Input: dimensioned drawing with shaded views. Units: mm. Origin: part minimum x, y, z. Give positions to 0.01 mm unless a question says otherwise; leave off trailing zeros. Loops run counter-clockwise (first coordinate to the right, second up) from the corner with the lowest first, then second, coordinate; pieces in that order, holes last.
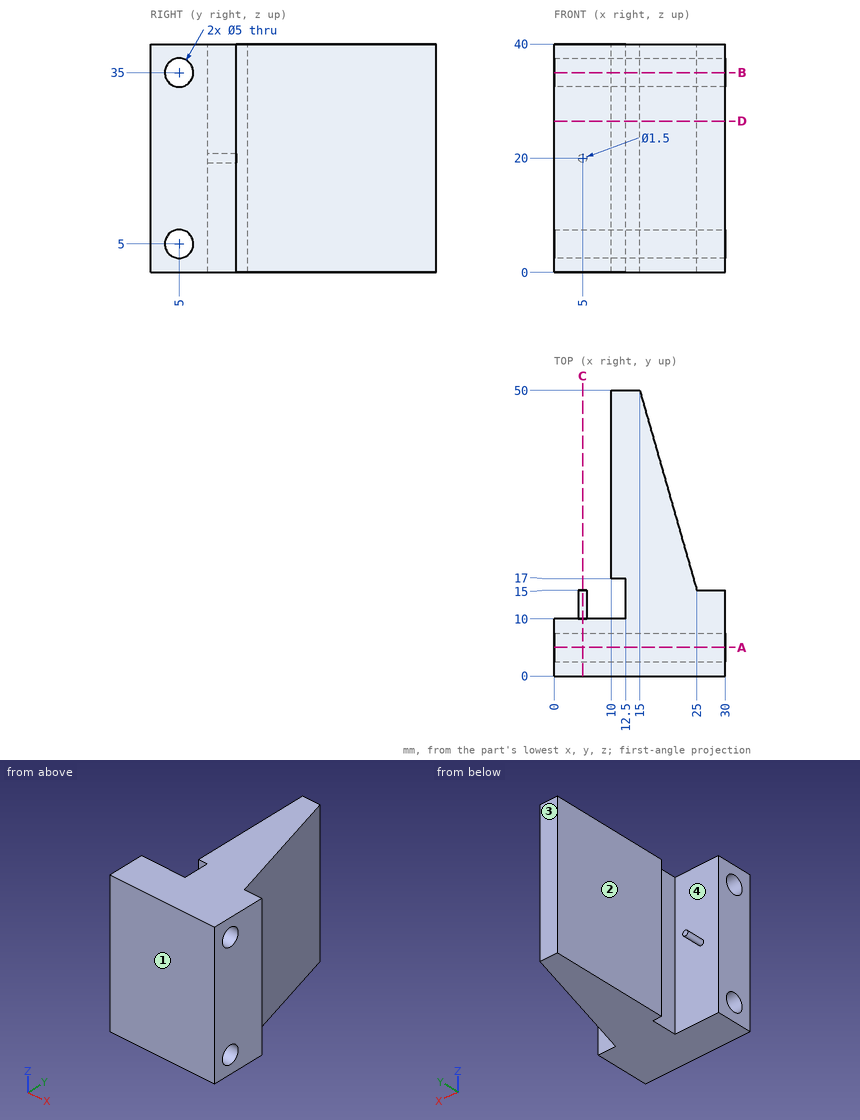
(1) Ray query, line 1 along Y through (x, z) = (10.25, 35); line 2 along Y through (x, z) = (14.25, 35); line 3 along Y through (x, z) = (3.5, 18). Return the intervals inside material, ascending.
A:
line 1: y = 0 to 2.5, 7.5 to 10, 17 to 50
line 2: y = 0 to 2.5, 7.5 to 50
line 3: y = 0 to 10
(2) Section D-D, the plane z = 26.5. Return the cut outline in (x, y).
A:
outline: (0, 0) - (30, 0) - (30, 15) - (25, 15) - (15, 50) - (10, 50) - (10, 17) - (12.5, 17) - (12.5, 10) - (0, 10) - close
(3) Section C-C, the plane x = 5. Return the cut outline in (y, z).
A:
outline: (0, 0) - (10, 0) - (10, 19.25) - (15, 19.25) - (15, 20.75) - (10, 20.75) - (10, 40) - (0, 40) - close; hole circle Ø5 at (5, 5); hole circle Ø5 at (5, 35)
(4) Section B-B, the plane z = 35. Return the cut outline in (x, y), then the cut area to 4 significant figures.
A:
outline: (0, 0) - (30, 0) - (30, 2.5) - (0, 2.5) - close; (0, 7.5) - (30, 7.5) - (30, 15) - (25, 15) - (15, 50) - (10, 50) - (10, 17) - (12.5, 17) - (12.5, 10) - (0, 10) - close
area: 582.5 mm2
(5) Section A-A, the plane y = 5. Return the cut outline in (x, z), then the cut area to 3 significant figures.
A:
outline: (0, 0) - (30, 0) - (30, 2.5) - (0, 2.5) - close; (0, 7.5) - (30, 7.5) - (30, 32.5) - (0, 32.5) - close; (0, 37.5) - (30, 37.5) - (30, 40) - (0, 40) - close
area: 900 mm2
(6) Mould query, pull axis Y, two halves, no side actions, for the marked faces 1, 2, 3 and 4. Classes: pulls with the +Y half, pulls with the -Y half, needs draft (parallel to the pull), parting line crosses it, or undercut.
A:
face 1: pulls with the -Y half
face 2: needs draft
face 3: pulls with the +Y half
face 4: undercut
(7) First-contact query: pin 1 (0.8 mm diameter, centred on x = 5, z = 20.5, fed in from +Y); pin 2 (2 mm diameter, centred on x = 7, z = 25.5, fed in from +Y). Flat tips, straight axial feed; report the tip coordinate or a pass-through.
A:
pin 1: stops at y = 15
pin 2: stops at y = 10
